The listing builds one solid part. Answer for the finished solid, in the listing's coordinates (mm). Face numbers are marked on the shaded views. A direction names the side the tool comes from. Give positions to 0.01 mm unless a question says otherwise; leave off trailing zeros. Order: outer loops, then holes, each group sorted by start corner. A loop starts at its lowest first (then second) coordinate and runs counter-clockwise, first axis right, second up. Notation, with made-up numbers: (69.5, 32.25) - (95.5, 32.25) arc R30 cw to (95.5, 70.25) - close; hole circle Ø2 at (50, 70). An arc over 180 degrees is marked (long way). Write each question's results on one line, items separated by ' | '. Start each with the question number.
1. Section C-C (z = 0.45) is taken. Give the vertices of the cut face in (x, y).
2. Find the intervals of material crossed by L1, parallel to X at y = -13, z = 0.3; L2, parallel to X at y = -4, z = 0.8; L3, parallel to Y at x = -14.5, z = 0.55, in increasing order.
3. Section A-A (x = 0) is taken. Give the vertices of the cut face in (y, z), and give its area (3 significant figures).
4. Section B-B (y = 0) is taken. Give the vertices of the cut face in (x, z).
5. A flat-ended cylindrical pin translates along its axis: pin 1 (1 mm diameter, centred on x = 0, y = -2, fed in from -Z). Find the tip coordinate at first contact, or state that the pin passes through.
6. Which of the six approach directions +Z, -Z, +X, -X, +Y, -Y give full straight-line access (tool end or side, diameter ignored) to the marked faces 1 and 2?
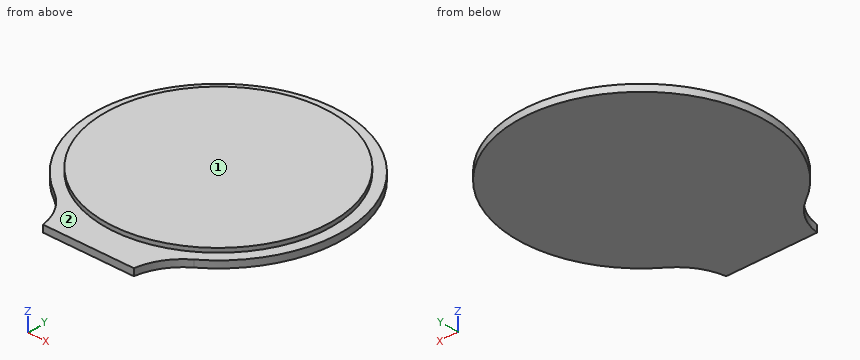
from build123d import *

# Parameters (mm, degrees)
BOSS_EXTRU_1_CONTOUR_CRAN_DEPTH = 1
CRAN_R                          = 16.256
BOSS_EXTRU_1_CRAN_DEPTH         = 0.6


with BuildPart() as part:
    # Contour_Écran → Boss.-Extru.1_Contour_Écran (new body)
    with BuildSketch(Plane.XY):
        with BuildLine():
            Line((-6.5, -20.3), (6.5, -20.3))
            ThreePointArc((6.5, -20.3), (7.668481961, -17.144005216), (10.005084126, -14.722034222))
            ThreePointArc((10.005084126, -14.722034222), (0, 17.8), (-10.005084126, -14.722034222))
            ThreePointArc((-10.005084126, -14.722034222), (-7.668481961, -17.144005216), (-6.5, -20.3))
        make_face()
    extrude(amount=BOSS_EXTRU_1_CONTOUR_CRAN_DEPTH)

    # cran → Boss.-Extru.1_Écran (add)
    with BuildSketch(Plane.XY.offset(1)):
        Circle(CRAN_R)
    extrude(amount=BOSS_EXTRU_1_CRAN_DEPTH)


solid = part.part
Reported:
1) outline: (-10.01, -14.72) arc R8.21 cw to (-6.5, -20.3) - (6.5, -20.3) arc R8.21 cw to (10.01, -14.72) arc R17.8 ccw (long way) to start
2) L1: -12.16 to 12.16 | L2: -17.34 to 17.34 | L3: -10.32 to 10.32
3) outline: (-20.3, 0) - (17.8, 0) - (17.8, 1) - (16.26, 1) - (16.26, 1.6) - (-16.26, 1.6) - (-16.26, 1) - (-20.3, 1) - close | area: 57.6 mm²
4) outline: (-17.8, 0) - (17.8, 0) - (17.8, 1) - (16.26, 1) - (16.26, 1.6) - (-16.26, 1.6) - (-16.26, 1) - (-17.8, 1) - close
5) pin 1: z = 0
6) face 1: +Z, +X, -X, +Y, -Y | face 2: +Z
